from build123d import *

# Parameters (mm, degrees)
SKETCH1_W           = 7.82
SKETCH1_H           = 51
BOSS_EXTRUDE1_DEPTH = 25
BOSS_EXTRUDE2_DEPTH = 5
BOSS_EXTRUDE3_DEPTH = 2
FILLET1_R           = 10
FILLET2_R           = 3
SKETCH4_W           = 3
SKETCH4_H           = 10
BOSS_EXTRUDE4_DEPTH = 2.5
CHAMFER1_SIZE       = 1


with BuildPart() as part:
    # Sketch1 → Boss-Extrude1 (new body)
    with BuildSketch(Plane(origin=(0, 0, 0), x_dir=(1, 0, 0), z_dir=(0, 1, 0))):
        Rectangle(SKETCH1_W, SKETCH1_H)
    extrude(amount=BOSS_EXTRUDE1_DEPTH)

    # Sketch2 → Boss-Extrude2 (add)
    with BuildSketch(Plane(origin=(0, 25, 0), x_dir=(1, 0, 0), z_dir=(0, 1, 0))):
        Polygon((-29.755356576, 1.98115624), (19.438138919, -22.615591532), (29.755356576, -1.98115624), (-19.438138919, 22.615591532), align=None)
    extrude(amount=BOSS_EXTRUDE2_DEPTH)

    # Sketch3 → Boss-Extrude3 (add)
    with BuildSketch(Plane(origin=(0, 30, 0), x_dir=(1, 0, 0), z_dir=(0, 1, 0))):
        Polygon((-29.755356576, 1.98115624), (19.438138919, -22.615591532), (29.755356576, -1.98115624), (-19.438138919, 22.615591532), align=None)
        Polygon((18.588433089, -20.066474038), (-27.206239081, 2.83086207), (-18.588433089, 20.066474038), (27.206239081, -2.83086207), align=None, mode=Mode.SUBTRACT)
    extrude(amount=BOSS_EXTRUDE3_DEPTH)

    # Fillet1
    fillet1_edges = [part.edges().sort_by_distance(p)[0] for p in [
        (-3.91, 25, -1.955000002),
    ]]
    fillet(fillet1_edges, radius=FILLET1_R)

    # Fillet2
    fillet2_edges = [part.edges().sort_by_distance(p)[0] for p in [
        (3.91, 25, 1.955000002),
    ]]
    fillet(fillet2_edges, radius=FILLET2_R)

    # Sketch4 → Boss-Extrude4 (add)
    with BuildSketch(Plane.ZY.offset(3.91)):
        Rectangle(SKETCH4_W, SKETCH4_H)
    extrude(amount=BOSS_EXTRUDE4_DEPTH)

    # Chamfer1
    chamfer1_edges = [part.edges().sort_by_distance(p)[0] for p in [
        (-3.91, 2.5, 1.5),
        (-3.91, 5, 0),
        (-3.91, 2.5, -1.5),
    ]]
    chamfer(chamfer1_edges, length=CHAMFER1_SIZE)


solid = part.part
The listing builds one solid part. Answer for the finished solid, in the listing's coordinates (mm). A direction names the side the tool comes from. Coordinates: 2 decimals unless noted, no trailing zeros. Loops run counter-clockwise (first coordinate to the right, second up) from the corner with the lowest first, then second, coordinate; pieces in that order, holes last. Notation, with made-up numbers: (59, -27.5) -> (75, -27.5) arc R5 ccw to (75, -23.5) -> close; hole circle Ø7 at (35, 8.25). An arc over 180 degrees is marked (long way). Answer in a Markdown table with one row per item. Add a question column.
1. Consider line 1 (Y direction, x = -24.5, z = -11); line 2 (Y direction, x = 12.5, z = 2); line 3 (X direction, y = 16, z = -20). Determine where each line is inside the solid, lowest interval first. Write a range as [from, to].
2. The part is cut by section B-B, the plane y = 1. Write down the section's boundary in (x, z).
3. The part is cut by section C-C, the plane x = 14. Write down the section's boundary in (y, z).
4. For faces 5 (the flat face through (-5, -1, -1.5)), 6 (the flat face through (-6, 5, 0)), 7 (the flat face through (16, 25, 6)), determine the directions among +Z, -Z, +X, -X, +Y, -Y from which every point of the face is accessible in a straight line to the end or side of a thin tool.
5. The part is cut by section A-A, the plane z = -16.5. Write down the section's boundary in (x, y), then the cut area to 3 significant figures.
6. Flat-ended cylindrical pins translate along their axes: P1, Ø0.9, axis at y = 1, z = -0.5, coming from the -X side; P2, Ø2.5, axis at y = -2, z = 0, coming from the +X side; P3, Ø5, axis at x = -8.5, z = 10, coming from the +Y side; P4, Ø8, axis at x = 10.5, z = -9.5, coming from the -Y side. Find the tip coordinate at first contact, or state that the pin passes through.
7. The part is cut by section D-D, the plane z = -8.5. Write down the section's boundary in (x, y).
8. Determine the mould class of faces 1 (the flat face through (24.525, 28.451, 12.443)), 2 (the flat face through (3.988, 30.986, -8.778)), 3 (the flat face through (22.958, 30.986, 11.328)), 4 (the flat face through (-5, -5, 0)) for opening direction Z: +Z half, -Z half, draft (parallel to the pull), parting line (faces both ways), or undercut.
Answer below:
| question | item | result |
|---|---|---|
| 1 | line 1 | [25, 32] |
| 1 | line 2 | [25, 30] |
| 1 | line 3 | [-3.91, 3.91] |
| 2 | outline | (-6.41, -1.5) -> (-4.91, -1.5) -> (-3.91, -2.5) -> (-3.91, -25.5) -> (3.91, -25.5) -> (3.91, 25.5) -> (-3.91, 25.5) -> (-3.91, 2.5) -> (-4.91, 1.5) -> (-6.41, 1.5) -> close |
| 3 | outline | (25, -5.9) -> (32, -5.9) -> (32, -3.77) -> (30, -3.77) -> (30, 17.77) -> (32, 17.77) -> (32, 19.9) -> (25, 19.9) -> close |
| 4 | face 5 | -Z, -X, -Y |
| 4 | face 6 | +Z, -Z, -X |
| 4 | face 7 | +Z, -Z, +X, -Y |
| 5 | outline | (-22.5, 25) -> (-13.91, 25) arc R10 cw to (-7.21, 22.42) -> (-7.21, 32) -> (-11.46, 32) -> (-11.46, 30) -> (-20.37, 30) -> (-20.37, 32) -> (-22.5, 32) -> close; (-3.91, 0) -> (3.91, 0) -> (3.91, 25) -> (-3.91, 25) -> close |
| 5 | area | 290 mm2 |
| 6 | P1 | x = -6.41 |
| 6 | P2 | x = -3.91 |
| 6 | P3 | y = 32 |
| 6 | P4 | y = 24.97 |
| 7 | outline | (-26.5, 25) -> (-13.91, 25) arc R10 cw to (-3.91, 15) -> (-3.91, 0) -> (3.91, 0) -> (3.91, 22) arc R3 cw to (6.91, 25) -> (8.79, 25) -> (8.79, 32) -> (4.54, 32) -> (4.54, 30) -> (-24.37, 30) -> (-24.37, 32) -> (-26.5, 32) -> close |
| 8 | face 1 | +Z half |
| 8 | face 2 | undercut |
| 8 | face 3 | undercut |
| 8 | face 4 | draft |
